Design review of the part built by this model. Coordinates are the model's own, in mm. A direction names the side the tool comes from. Round coordinates to 2 decimals unless told otherwise and drop trailing zeros. Write each loop counter-clockwise with the first axis right and the second up, starting at its lowest first coordinate (ties: lowest second). Pieces come first, ordered by that corner, then holes. Notation, with made-up numbers: (49, 72) - (66, 72) arc R21 cw to (66, 83) - close; hole circle Ø3 at (82, -39.75). An arc over 180 degrees is marked (long way). Use one line per item in the form item = value.
Autodesk Inventor part; units mm, degrees
ref_plane "YZ Plane" through (0, 0, 0) normal (1, 0, 0) x (0, 1, 0)
ref_plane "XZ Plane" through (0, 0, 0) normal (0, 1, 0) x (-1, 0, 0)
ref_plane "XY Plane" through (0, 0, 0) normal (0, 0, 1) x (1, 0, 0)
sketch "スケッチ1" plane through (0, 0, 0) normal (1, 0, 0) x (0, 1, 0)
  line L0 (5, 5) -> (-5, 5)
  line L1 (-5, 5) -> (-5, -5)
  line L2 (-5, -5) -> (5, -5)
  line L3 (5, -5) -> (5, 5)
  line L4 (4, 4) -> (-4, 4)
  line L5 (-4, 4) -> (-4, -4)
  line L6 (-4, -4) -> (4, -4)
  line L7 (4, -4) -> (4, 4)
  point P0 (0, 0)
  dimension "d0" = 1
  dimension "d1" = 1
  dimension "d2" = 1
  dimension "d3" = 1
  dimension "d4" = 10
  dimension "d5" = 10
  dimension "d6" = 5
  dimension "d7" = 5
extrude "押し出し1" add sketch "スケッチ1" along normal blind 240
sketch "スケッチ2" plane through (0, -5, 5) normal (0, 0, 1) x (1, 0, 0)
  circle A0 centre (5, 5) radius 1.5
  circle A1 centre (235, 5) radius 1.5
  line L0 (240, 10) -> (240, 0)
  line L1 (0, 0) -> (240, 0)
  line L2 (0, 10) -> (0, 0)
  point P0 (0, 5)
  dimension "d10" = 5
  dimension "d11" = 3
  dimension "d12" = 5
  dimension "d13" = 5
  dimension "d14" = 5
  dimension "d15" = 3
extrude "押し出し2" cut sketch "スケッチ2" against normal blind 230
sketch "スケッチ3" plane through (0, -5, -5) normal (0, -1, 0) x (1, 0, 0)
  circle A0 centre (15, 5) radius 1.5
  line L0 (0, 10) -> (0, 0)
  circle A1 centre (225, 5) radius 1.5
  line L1 (240, 10) -> (240, 0)
  line L2 (0, 0) -> (240, 0)
  point P0 (0, 5)
  dimension "d18" = 3
  dimension "d19" = 15
  dimension "d20" = 3
  dimension "d21" = 15
  dimension "d22" = 5
  dimension "d23" = 5
extrude "押し出し3" cut sketch "スケッチ3" against normal blind 230
properties part number "sideparts" material "アルミニウム 6061"
Q1. We need section A-A on y = 0. Write out the cut boundary in (x, z).
Calculated:
outline = (0, -5) - (3.5, -5) - (3.5, -4) - (0, -4) - close; (0, 4) - (3.5, 4) - (3.5, 5) - (0, 5) - close; (6.5, -5) - (233.5, -5) - (233.5, -4) - (6.5, -4) - close; (6.5, 4) - (233.5, 4) - (233.5, 5) - (6.5, 5) - close; (236.5, -5) - (240, -5) - (240, -4) - (236.5, -4) - close; (236.5, 4) - (240, 4) - (240, 5) - (236.5, 5) - close
Q2. Draft analysis for pull direction Y (two halves, no side actions). For faces 1 (the flat face through (240, -4.5, 0.1)), 2 (the flat face through (118, 0, -4)), 3 (the flat face through (118, 5, 0)), state which applies: released by +Y, released by -Y, zero draft, split by the parting line, or undercut.
Calculated:
face_1 = zero draft
face_2 = undercut
face_3 = released by +Y
Q3. We need section C-C on x = 47.5. Write out the cut boundary in (y, z).
Calculated:
outline = (-5, -5) - (5, -5) - (5, 5) - (-5, 5) - close; hole (-4, -4) - (4, -4) - (4, 4) - (-4, 4) - close
Q4. To check wall thickness, follow line 1 along Y through (x, z) = (85, 0.25); line 2 along Y through (x, z) = (235, 4.8). State the ranges of each line that lie inside material, in increasing order. Write a range as from..to.
Calculated:
line_1 = -5..-4, 4..5
line_2 = -5..-1.5, 1.5..5
Q5. We need section B-B on z = 0. Write out the cut boundary in (x, y).
Calculated:
outline = (0, -5) - (13.5, -5) - (13.5, -4) - (0, -4) - close; (0, 4) - (13.5, 4) - (13.5, 5) - (0, 5) - close; (16.5, -5) - (223.5, -5) - (223.5, -4) - (16.5, -4) - close; (16.5, 4) - (223.5, 4) - (223.5, 5) - (16.5, 5) - close; (226.5, -5) - (240, -5) - (240, -4) - (226.5, -4) - close; (226.5, 4) - (240, 4) - (240, 5) - (226.5, 5) - close
Q6. For P1, Ø1.8, axis at x = 5, y = 0, coming from the -Z side; P2, Ø3.5, axis at x = 15, z = 0, coming from the +Y side, all flat-tipped, find the tip position at first contact; note any pin that passes through.
Calculated:
P1 = through
P2 = 5
Q7. Machinability: for faces 4 (the flat face through (118, 0, -5)), 5 (the flat face through (118, 4, 0)), which of the approach directions +Z, -Z, +X, -X, +Y, -Y give a long, thin tool a straight path to every point of the face, cutting with its end or side? Answer none if there is none.
Calculated:
face_4 = -Z, +X, -X, +Y, -Y
face_5 = +X, -X
